Geometry: final body of the model. Coordinates: model frame, mm. A direction names the side the tool comes from. Give positions to 0.01 mm unless a question says otherwise; leave off trailing zeros. Order: outer loops, then holes, each group sorted by start corner. A loop starts at its lowest first (then second) coordinate and runs counter-clockwise, first axis right, second up. Notation, with made-up numbers: (-2.75, 77.5) -> (33.25, 77.5) arc R19 ccw to (33.25, 95.5) -> close; hole circle Ø7 at (-25, 45.25). An arc over 180 degrees is marked (long way). One line per question, with ' | ' between items. Start each with the question number.
(1) Section B-B (y = 10). Return loops of the section in (x, z).
(2) Ray query, L1, parallel to Y at x = 0, z = 19; L2, parallel to X at y = 0, z = 25.5; L3, parallel to Z at x = 4.5, y = 5. Return the intervals inside material, ascending.
(3) Set-up query: faces 1 (the face through (6, 0, 42)), 2 (the face through (0.171, 6.337, 10.775)). Return all of +Z, -Z, +X, -X, +Y, -Y with unobstructed straight access to the full face (end or side cutting, diameter ignored); none if empty.
(4) First-contact query: pin 1 Ø6 at (x, z) = (-4, 9.5) entering from +Y; pin 2 Ø1 at (x, z) = (-3.5, 7) entering from +Y; pin 3 Ø1.5 at (x, z) = (-7.5, -25.5) entering from -Y. Flat tips, straight axial feed; report the tip coordinate or a pass-through.
(5) Section A-A (x = 0). Return loops of the section in (y, z).
(6) Section C-C (y = -1.5). Return loops of the section in (x, z), then the cut area to 3 significant figures.
(7) Mould query, pull axis X, two halves, no side actions, for faces 3 (the face through (-1.08, -4.88, 26.96)), 4 (the face through (-5, 0, -27)), 5 (the face through (-12.247, 0, -24)), 6 (the face through (0, 12.5, 0)). Classes: +X half, -X half, draft (parallel to the pull), parting line (faces both ways), or undercut.
(8) Section D-D (z = 32.5). Return loops of the section in (x, y), then the cut area to 3 significant figures.
```python
from build123d import *

# Parameters (mm, degrees)
SKETCH1_R           = 17.5
BOSS_EXTRUDE1_DEPTH = 42
SKETCH3_W           = 21.176447949
SKETCH3_H           = 25
CUT_EXTRUDE1_DEPTH  = 88.569972022
SKETCH4_R           = 5
CUT_EXTRUDE2_DEPTH  = 87.67323693
CUT_EXTRUDE3_DEPTH  = 74


with BuildPart() as part:
    # Sketch1 → Boss-Extrude1 (new, symmetric)
    with BuildSketch(Plane.XY):
        with Locations(Location((0, 0, 0), (0, 0, 180))):
            Circle(SKETCH1_R)
    extrude(amount=BOSS_EXTRUDE1_DEPTH, both=True)

    # Sketch3 → Cut-Extrude1 (cut, through all)
    with BuildSketch(Plane.XY.offset(42)):
        with Locations((-22.835672689, 0)):
            Rectangle(SKETCH3_W, SKETCH3_H)
        with Locations((22.835672689, 0)):
            Rectangle(SKETCH3_W, SKETCH3_H)
    extrude(amount=-CUT_EXTRUDE1_DEPTH, mode=Mode.SUBTRACT)

    # Sketch4 → Cut-Extrude2 (cut, through all)
    with BuildSketch(Plane.XY.offset(42)):
        Circle(SKETCH4_R)
    extrude(amount=-CUT_EXTRUDE2_DEPTH, mode=Mode.SUBTRACT)

    # Sketch5 → Cut-Extrude3 (cut)
    with BuildSketch(Plane(origin=(12.247448714, 0, 0), x_dir=(0, 0, -1), z_dir=(1, 0, 0))):
        Polygon((14.43375673, 0), (7.216878365, 12.5), (-7.216878365, 12.5), (-14.43375673, 0), (-7.216878365, -12.5), (7.216878365, -12.5), align=None)
    extrude(amount=-CUT_EXTRUDE3_DEPTH, mode=Mode.SUBTRACT)


solid = part.part
```
Response:
1) outline: (-12.25, -42) -> (12.25, -42) -> (12.25, -8.66) -> (-12.25, -8.66) -> close; (-12.25, 8.66) -> (12.25, 8.66) -> (12.25, 42) -> (-12.25, 42) -> close
2) L1: y = -17.5 to -5, 5 to 17.5 | L2: x = -12.25 to -5, 5 to 12.25 | L3: z = -42 to -11.55, 11.55 to 42
3) face 1: +Z, +X, -X, +Y, -Y | face 2: +X, -X
4) pin 1: stops at y = 17.47 | pin 2: stops at y = 17.24 | pin 3: stops at y = -16.15
5) outline: (-17.5, -42) -> (-5, -42) -> (-5, -11.55) -> (-12.5, -7.22) -> (-12.5, 7.22) -> (-5, 11.55) -> (-5, 42) -> (-17.5, 42) -> close; (5, -42) -> (17.5, -42) -> (17.5, 42) -> (5, 42) -> (5, 11.55) -> (12.5, 7.22) -> (12.5, -7.22) -> (5, -11.55) -> close
6) outline: (-12.25, -42) -> (-4.77, -42) -> (-4.77, -13.57) -> (-12.25, -13.57) -> close; (-12.25, 13.57) -> (-4.77, 13.57) -> (-4.77, 42) -> (-12.25, 42) -> close; (4.77, -42) -> (12.25, -42) -> (12.25, -13.57) -> (4.77, -13.57) -> close; (4.77, 13.57) -> (12.25, 13.57) -> (12.25, 42) -> (4.77, 42) -> close | area: 850 mm^2
7) face 3: undercut | face 4: undercut | face 5: -X half | face 6: draft
8) outline: (-12.25, -12.5) arc R17.5 ccw to (12.25, -12.5) -> (12.25, 12.5) arc R17.5 ccw to (-12.25, 12.5) -> close; hole circle Ø10 at (0, 0) | area: 702 mm^2
